Verification items for the finished model (mm, model axes). Face numbers are marked on the shaded views. A direction names the side the tool comes from. Coordinates: 2 decimals unless noted, no trailing zeros. Order: outer loops, then holes, each group sorted by start corner. A loop starts at its lowest first (then second) coordinate and runs counter-clockwise, first axis right, second up. Notation, with made-up numbers: M 10,12.5 L 25,12.5 A19 cw 25,30.5 Z; hole C 56,-35 d3. An arc over 180 degrees is marked long. Write item = value, one per line.
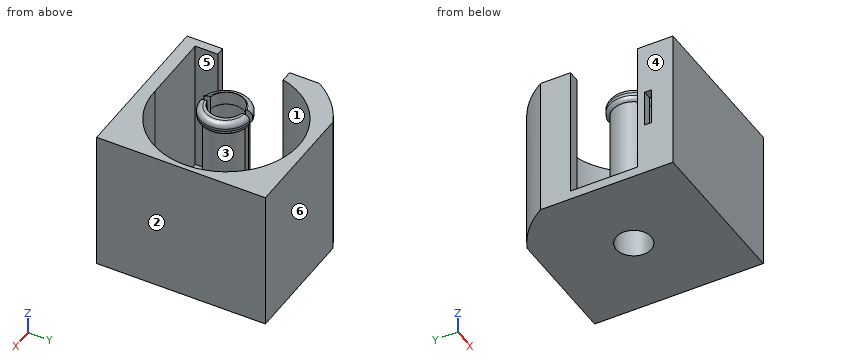
```python
from build123d import *

# Parameters (mm, degrees)
F0_R      = 7.9
F1_DEPTH  = 4
F2_R      = 9.4
F2_R_2    = 7.9
F3_DEPTH  = 60
F4_W      = 3.080128
F4_H      = 16.594132
F5_DEPTH  = 25
F6_R      = 11.341969
F6_R_2    = 7.956315
F7_DEPTH  = 6
F8_R      = 2.5
F9_W      = 2.779254
F9_H      = 27.416152
F10_DEPTH = 40


with BuildPart() as f1:
    # F0 (on Top) → F1 (new body)
    with BuildSketch(Plane.XY):
        with BuildLine():
            Line((36, 38), (-17.888544, 38))
            ThreePointArc((-17.888544, 38), (-28.159562, 31.1615), (-36, 21.633308))
            Line((-36, 21.633308), (-36, -38))
            Line((-36, -38), (36, -38))
            Line((36, -38), (36, 38))
        make_face()
        Circle(F0_R, mode=Mode.SUBTRACT)
    extrude(amount=F1_DEPTH)

    # F2 (on face) → F3 (join)
    with BuildSketch(Plane.XY.offset(4)):
        Circle(F2_R)
        Circle(F2_R_2, mode=Mode.SUBTRACT)
        with BuildLine():
            Line((36, 38), (-17.888544, 38))
            ThreePointArc((-17.888544, 38), (-28.159562, 31.1615), (-36, 21.633308))
            Line((-36, 21.633308), (-36, 8.167186))
            Line((-36, 8.167186), (-30.917966, 8.167186))
            ThreePointArc((-30.917966, 8.167186), (27.040261, 20.60372), (0, -32.147087))
            Line((0, -32.147087), (-32.136563, -32.147087))
            Line((-32.136563, -32.147087), (-32.136563, -29.065894))
            Line((-32.136563, -29.065894), (-32.136563, -21.989353))
            Line((-32.136563, -21.989353), (-36, -21.989353))
            Line((-36, -21.989353), (-36, -29.065894))
            Line((-36, -29.065894), (-36, -38))
            Line((-36, -38), (36, -38))
            Line((36, -38), (36, 38))
        make_face()
    extrude(amount=F3_DEPTH)

    # F4 (on face) → F5 (cut)
    with BuildSketch(Plane(origin=(-36, 0, 0), x_dir=(0, -1, 0), z_dir=(-1, 0, 0))):
        with Locations((26.73703, 32.321629)):
            Rectangle(F4_W, F4_H)
    extrude(amount=-F5_DEPTH, mode=Mode.SUBTRACT)

    # F6 (on face) → F7 (join)
    with BuildSketch(Plane.XY.offset(64)):
        with Locations((0.724832, 0)):
            Circle(F6_R)
        Circle(F6_R_2, mode=Mode.SUBTRACT)
    extrude(amount=F7_DEPTH)

    # F8
    f8_edges = [f1.edges().sort_by_distance(p)[0] for p in [
        (-10.617137, 0, 70),
        (-10.617137, 0, 64),
    ]]
    fillet(f8_edges, radius=F8_R)

    # F9 (on face) → F10 (cut)
    with BuildSketch(Plane.XY.offset(70)):
        Rectangle(F9_W, F9_H)
    extrude(amount=-F10_DEPTH, mode=Mode.SUBTRACT)


solid = f1.part
```
Item 1: Sectioned sample at A-A, the plane z = 12. Enter the section's corners in (x, y), then the cut area to 3 significant figures.
Report:
outline = M -36,-38 L 36,-38 L 36,38 L -17.89,38 A42 ccw -36,21.63 L -36,8.17 L -30.92,8.17 A32.8 cw long 0,-32.15 L -32.14,-32.15 L -32.14,-21.99 L -36,-21.99 Z; C 0,0 d18.8; hole C 0,0 d15.8
area = 1,690 mm^2
Item 2: Sectioned sample at D-D, the plane z = 46.5. Enter the section's corners in (x, y).
Report:
outline = M -36,-38 L 36,-38 L 36,38 L -17.89,38 A42 ccw -36,21.63 L -36,8.17 L -30.92,8.17 A32.8 cw long 0,-32.15 L -32.14,-32.15 L -32.14,-21.99 L -36,-21.99 Z; M -1.39,-9.3 L -1.39,-7.78 A7.9 cw -1.39,7.78 L -1.39,9.3 A9.4 ccw Z; M 1.39,-9.3 A9.4 ccw 1.39,9.3 L 1.39,7.78 A7.9 cw 1.39,-7.78 Z
Item 3: Sectioned sample at B-B, the plane z = 28.5. Enter the section's corners in (x, y).
Report:
outline = M -36,-38 L 36,-38 L 36,38 L -17.89,38 A42 ccw -36,21.63 L -36,8.17 L -30.92,8.17 A32.8 cw long 0,-32.15 L -32.14,-32.15 L -32.14,-28.28 L -36,-28.28 Z; M -36,-25.2 L -32.14,-25.2 L -32.14,-21.99 L -36,-21.99 Z; C 0,0 d18.8; hole C 0,0 d15.8
Item 4: Release check for a two-part mould opening along X. For the marked faces 1, 2, 3 and 4 record: pulls with the +X half, pulls with the -X half, needs draft (parallel to the pull), parting line crosses it, or undercut.
Report:
face_1 = undercut
face_2 = pulls with the +X half
face_3 = undercut
face_4 = pulls with the -X half
Item 5: Tool access check on the marked faces 5 and 6. Record the directions out of +Z, -Z, +X, -X, +Y, -Y that give a thin tool (end or side, any length) a straight path to the whole face; none if there is none.
Report:
face_5 = +Z
face_6 = +Z, -Z, +X, -X, +Y
Item 6: Gauge pin test, flat ends, axial feed: pin 1 (1.2 mm diameter, centred on x = -35, z = 45, fed in from +Y); pin 2 (10 mm diameter, centred on x = 24.5, y = 10.5, fed in from +Z); pin 3 (3 mm diameter, centred on x = -33.5, z = 34.5, fed in from +Y). Record the tip position at first contact, or that the pin passes through.
Report:
pin_1 = 24.1
pin_2 = 4
pin_3 = 27.2
Item 7: Scan lines: L1, parallel to Y at x = -3, z = 31; L2, parallel to X at y = 0, z = 37; L3, parallel to Y at x = 2, z = 63. Record each from-to range of solid material in increasing order. Write a range as from..to.
Report:
L1 = -38..-32.15, -8.91..-7.31, 7.31..8.91, 33.2..38
L2 = -9.4..-7.9, 7.9..9.4, 33.81..36
L3 = -38..-32.15, -9.18..-7.64, 7.64..9.18, 33.43..38
Item 8: Sectioned sample at C-C, the plane x = 25. Enter the section's corners in (y, z).
Report:
outline = M -38,0 L 38,0 L 38,64 L 23.01,64 L 23.01,4 L -21.73,4 L -21.73,64 L -38,64 Z
